Design review of the part built by this model. Coordinates are the model's own, in mm. Face numbers are marked on the shaded views. A direction names the side the tool comes from. Coordinates: 2 decimals unless noted, no trailing zeros. Write each loop counter-clockwise with the first axis right and the second up, starting at its lowest first coordinate (ties: lowest second). Pieces come first, ordered by that corner, then holes. Notation, with made-up numbers: (25, 13) -> (42, 13) arc R19 ccw to (42, 45) -> close; hole circle Ø2 at (25, 70.25). An arc over 180 degrees is marked (long way). Answer in a Markdown table with one row per item. Add a question column.
Item 1: Take a section at B-B, the plane x = 0. Write out the cut boundary in (y, z) (3 decimals), and give its area (3 significant figures).
Item 2: Take a section at D-D, the plane x = 2.5. Write out the cut boundary in (y, z).
Item 3: Take a section at C-C, the plane z = 2.75. Give the number of separate pieces and of enclosed holes in the cut face, and give its area (3 significant figures).
Item 4: For the marked faces 4 and 5, list the 3-axis set-ups (+Z, -Z, +X, -X, +Y, -Y) from which the entire face can be reached by the end or side of a thin tool; tool diameter is ignored.
Item 5: Clearance check with a flat-ended pin moving along its axis: P1, Ø0.5, axis at x = 3.5, y = 0.5, coming from the +Z side. State where the tip first meets the part, or that it passes through.
Item 6: Draft analysis for pull direction X (two halves, no side actions). For the marked faces 1, 2 and 3, state which applies: released by +X, released by -X, zero draft, split by the parting line, or undercut.
Item 7: Take a section at A-A, the plane y = 0. Write out the cut boundary in (x, z), and give its area (3 significant figures).
Item 8: To check wall thickness, follow line 1 (Y direction, x = -2.5, z = 2.55); line 2 (Y direction, x = -1, z = 2.2); line 3 (X direction, y = 3.75, z = 2.2). State the ranges of each line that lie inside material, in increasing order.
from build123d import *

# Parameters (mm, degrees)
SZKIC1_R                    = 4.5
SZKIC1_R_2                  = 0.5
DODANIE_WYCI_GNI_CIE1_DEPTH = 3
SZKIC2_R                    = 0.5
WYTNIJ_WYCI_GNI_CIE2_DEPTH  = 1


with BuildPart() as part:
    # Szkic1 → Dodanie-wyciągnięcie1 (new body)
    with BuildSketch(Plane.XY):
        Circle(SZKIC1_R)
        Circle(SZKIC1_R_2, mode=Mode.SUBTRACT)
    extrude(amount=DODANIE_WYCI_GNI_CIE1_DEPTH)

    # Szkic2 → Wytnij-wyciągnięcie2 (cut)
    with BuildSketch(Plane.XY.offset(3)):
        with Locations((0, 3.625)):
            Circle(SZKIC2_R)
        with Locations((1.23982302, 3.40638575)):
            Circle(SZKIC2_R)
        with Locations((2.330105085, 2.776911106)):
            Circle(SZKIC2_R)
        with Locations((3.139342089, 1.8125)):
            Circle(SZKIC2_R)
        with Locations((3.569928105, 0.629474644)):
            Circle(SZKIC2_R)
        with Locations((3.569928105, -0.629474644)):
            Circle(SZKIC2_R)
        with Locations((3.139342089, -1.8125)):
            Circle(SZKIC2_R)
        with Locations((2.330105085, -2.776911106)):
            Circle(SZKIC2_R)
        with Locations((1.23982302, -3.40638575)):
            Circle(SZKIC2_R)
        with Locations((0, -3.625)):
            Circle(SZKIC2_R)
        with Locations((-1.23982302, -3.40638575)):
            Circle(SZKIC2_R)
        with Locations((-2.330105085, -2.776911106)):
            Circle(SZKIC2_R)
        with Locations((-3.139342089, -1.8125)):
            Circle(SZKIC2_R)
        with Locations((-3.569928105, -0.629474644)):
            Circle(SZKIC2_R)
        with Locations((-3.569928105, 0.629474644)):
            Circle(SZKIC2_R)
        with Locations((-3.139342089, 1.8125)):
            Circle(SZKIC2_R)
        with Locations((-2.330105085, 2.776911106)):
            Circle(SZKIC2_R)
        with Locations((-1.23982302, 3.40638575)):
            Circle(SZKIC2_R)
    extrude(amount=-WYTNIJ_WYCI_GNI_CIE2_DEPTH, mode=Mode.SUBTRACT)


solid = part.part
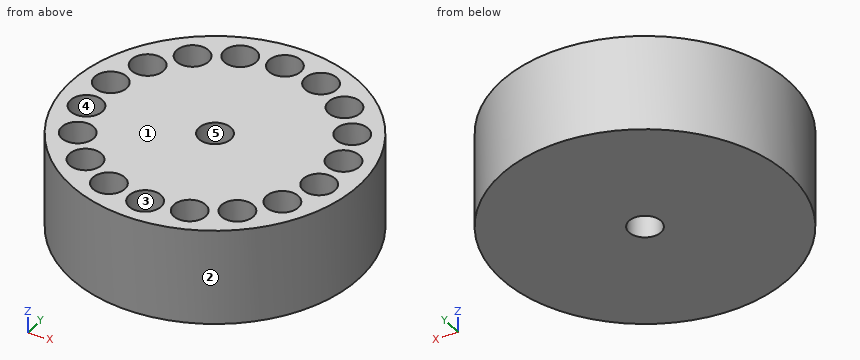
Answers:
| question | item | result |
|---|---|---|
| 1 | outline | (-4.5, 0) -> (-0.5, 0) -> (-0.5, 3) -> (-3.125, 3) -> (-3.125, 2) -> (-4.125, 2) -> (-4.125, 3) -> (-4.5, 3) -> close; (0.5, 0) -> (4.5, 0) -> (4.5, 3) -> (4.125, 3) -> (4.125, 2) -> (3.125, 2) -> (3.125, 3) -> (0.5, 3) -> close |
| 1 | area | 22.0 mm^2 |
| 2 | outline | (-3.74, 0) -> (3.74, 0) -> (3.74, 3) -> (3.25, 3) -> (3.25, 2) -> (2.31, 2) -> (2.31, 3) -> (-2.31, 3) -> (-2.31, 2) -> (-3.25, 2) -> (-3.25, 3) -> (-3.74, 3) -> close |
| 3 | separate pieces | 1 |
| 3 | enclosed holes | 19 |
| 3 | area | 48.7 mm^2 |
| 4 | face 4 | +Z |
| 4 | face 5 | +Z, -Z |
| 5 | P1 | stops at z = 2 |
| 6 | face 1 | zero draft |
| 6 | face 2 | split by the parting line |
| 6 | face 3 | undercut |
| 7 | outline | (-4.5, 0) -> (-0.5, 0) -> (-0.5, 3) -> (-4.5, 3) -> close; (0.5, 0) -> (4.5, 0) -> (4.5, 3) -> (0.5, 3) -> close |
| 7 | area | 24.0 mm^2 |
| 8 | line 1 | y = -3.74 to -3.25, -2.31 to 2.31, 3.25 to 3.74 |
| 8 | line 2 | y = -4.39 to -3.85, -2.97 to 2.97, 3.85 to 4.39 |
| 8 | line 3 | x = -2.49 to -1.6, -0.88 to -0.48, 0.48 to 0.88, 1.6 to 2.49 |
